Work out the finished part from the listing and answer in its coordinate system (mm). A direction names the side the tool comes from. Coordinates: 2 decimals unless noted, no trailing zeros. Write each loop counter-clockwise with the first axis right and the second up, starting at its lowest first coordinate (ties: lowest second). Pieces come first, ordered by that corner, then holes. Notation, with made-up numbers: (23, 5.5) - (31, 5.5) arc R12 cw to (31, 21.5) - close; hole circle Ø5 at (48, -19). An arc over 180 degrees is marked (long way). Use one line per item in the form item = value. Start each with the question number.
Item 1: A cutting plane is placed at A-A (y = 0). Write down the section's boundary in (x, z).
Item 2: Given pin 1 (5 mm diameter, centred on x = 5.5, z = 22.5, fed in from -Y); pin 2 (1.8 mm diameter, centred on x = -4.24, y = -4.24, fed in from -Z); pin 3 (5 mm diameter, centred on y = 3.5, z = 14.5, fed in from +X); pin 4 (5 mm diameter, centred on y = 1.5, z = 19, fed in from -X), each flat-ended and moving along its own axis, determine where each tip first touches the part or whether it passes through.
Item 3: A cutting plane is placed at B-B (x = 0). Write down the section's boundary in (y, z).
Item 4: A cutting plane is placed at C-C (z = 1). Write down the section's boundary in (x, y), then the cut area to 3 significant figures.
Item 5: Consider probe 1 along Z at (x, y) = (-6.5, 4.5); probe 2 along Y at (x, z) = (4.75, 12); probe 3 along Y at (x, z) = (6.5, 3.5). Determine where each line is inside the solid, lowest interval first.
Item 6: For faces 5 (the flat face through (0, 0, 30.5)), 6 (the cylindrical face through (-3.506, 3.567, 1.014)), 7 (the flat face through (2, -2, 18.5)), determine the directions among +Z, -Z, +X, -X, +Y, -Y from which every point of the face is accessible in a straight line to the end or side of a thin tool.
Item 7: A cutting plane is placed at D-D (z = 17). Write down the section's boundary in (x, y).
Item 8: Determine the mould class of faces 1 (the cylindrical face through (-0.54, -2.44, 24.42)), 2 (the conical face through (-4.38, -4.14, 2.5)), 3 (the flat face through (2, -2, 0)), 4 (the cylindrical face through (5.24, 4.2, 1.01)) for opening direction Y: released by +Y, released by -Y, zero draft, split by the parting line, or undercut.
from build123d import *

# Parameters (mm, degrees)
F0_R      = 9.3
F4_DEPTH  = 18.5
F2_R      = 2.5
F5_DEPTH  = 30.5
F3_R      = 2
F6_DEPTH  = 1.75
F7_SIZE2  = 1.3
F7_SIZE   = 5
F8_R      = 1
F9_DEPTH  = 20
F10_D     = 2
F10_DEPTH = 2
F10_TIP   = 0.600860619


with BuildPart() as f4:
    # F0 (on Top) → F4 (new body)
    with BuildSketch(Plane.XY):
        Circle(F0_R)
    extrude(amount=F4_DEPTH)

    # F2 (on Top) → F5 (join)
    with BuildSketch(Plane.XY):
        Circle(F2_R)
    extrude(amount=F5_DEPTH)

    # F3 (on Top) → F6 (join)
    with BuildSketch(Plane.XY):
        Circle(F3_R)
    extrude(amount=-F6_DEPTH)

    # F7
    f7_edges = [f4.edges().sort_by_distance(p)[0] for p in [
        (-9.3, 0, 0),
    ]]
    f7_side = f4.faces().sort_by_distance((-9.3, 0, 9.25))[0]
    chamfer(f7_edges, length=F7_SIZE, length2=F7_SIZE2, reference=f7_side)

    # F8 (on Right) → F9 (join)
    with BuildSketch(Plane.YZ):
        with Locations((0, 2.5)):
            Circle(F8_R)
        with Locations((-3, 2.5)):
            Circle(F8_R)
        with Locations((3, 2.5)):
            Circle(F8_R)
    extrude(amount=-F9_DEPTH)

    # F10
    with Locations(Plane(origin=(0, 0, 0), x_dir=(1, 0, 0), z_dir=(0, 0, -1))):
        with Locations((-4.2426406871, -4.2426406871), (-4.2426406871, 4.2426406871), (4.2426406871, 4.2426406871), (4.2426406871, -4.2426406871)):
            Hole(F10_D / 2, depth=F10_DEPTH)
            with Locations((0, 0, -(F10_DEPTH + F10_TIP / 2))):  # 118° drill point
                Cone(0, F10_D / 2, F10_TIP, mode=Mode.SUBTRACT)


solid = f4.part
Answer:
q1.outline = (-20, 1.5) - (-8.39, 1.5) - (-8, 0) - (-2, 0) - (-2, -1.75) - (2, -1.75) - (2, 0) - (8, 0) - (9.3, 5) - (9.3, 18.5) - (2.5, 18.5) - (2.5, 30.5) - (-2.5, 30.5) - (-2.5, 18.5) - (-9.3, 18.5) - (-9.3, 5) - (-8.91, 3.5) - (-20, 3.5) - close
q2.pin_1 = through
q2.pin_2 = 2.06
q2.pin_3 = 9.25
q2.pin_4 = -9.3
q3.outline = (-9.3, 5) - (-8, 0) - (-2, 0) - (-2, -1.75) - (2, -1.75) - (2, 0) - (8, 0) - (9.3, 5) - (9.3, 18.5) - (2.5, 18.5) - (2.5, 30.5) - (-2.5, 30.5) - (-2.5, 18.5) - (-9.3, 18.5) - close
q4.outline = circle Ø16.52 at (0, 0); hole circle Ø2 at (-4.24, -4.24); hole circle Ø2 at (-4.24, 4.24); hole circle Ø2 at (4.24, -4.24); hole circle Ø2 at (4.24, 4.24)
q4.area = 202 mm²
q5.probe_1 = 0 to 18.5
q5.probe_2 = -8 to 8
q5.probe_3 = -6.09 to 6.09
q6.face_5 = +Z, +X, -X, +Y, -Y
q6.face_6 = -Z
q6.face_7 = +Z
q7.outline = circle Ø18.6 at (0, 0)
q8.face_1 = split by the parting line
q8.face_2 = undercut
q8.face_3 = zero draft
q8.face_4 = undercut
